For this review, take the finished solid that the model builds, in its own axes (mm). Round coordinates to 2 decimals unless told otherwise and drop trailing zeros. Order: outer loops, then holes, each group sorted by start corner. A loop starts at its lowest first (then second) coordinate and runs counter-clockwise, first axis right, second up.
```python
from build123d import *

# Parameters (mm, degrees)
F1_DEPTH = 3
F2_D     = 3.3
F3_D     = 4.3
F4_R     = 5


# Not quite as in the source:
# - a feature names something its author has since deleted; it is built from what else it names


with BuildPart() as f1:
    # F0 (on Top) → F1 (new body)
    with BuildSketch(Plane.XY):
        Polygon((-43.9476147294, -54.0188625455), (24.4538411498, -54.0188625455), (24.4538411498, 61.4031404257), (-43.9476147294, 61.4031404257), (-43.9476147294, 45.1967306435), align=None)
    extrude(amount=F1_DEPTH)

    # F2 (through all)
    with Locations(Plane(origin=(0, 0, 0), x_dir=(1, 0, 0), z_dir=(0, 0, -1))):
        with Locations((-37.0104938323, -45.9071589798), (11.4895061677, -52.6071589798), (11.4895061677, 30.2928410202), (-37.0104938323, 28.9928410202)):
            Hole(F2_D / 2)

    # F3 (through all)
    with Locations(Plane(origin=(0, 0, 0), x_dir=(1, 0, 0), z_dir=(0, 0, -1))):
        with Locations((-21.5, -46.5), (21.5, -46.5), (21.5, 46.5), (-21.5, 46.5)):
            Hole(F3_D / 2)

    # F4
    f4_edges = [f1.edges().sort_by_distance(p)[0] for p in [
        (-43.947615, -54.018863, 1.5),
        (24.453841, -54.018863, 1.5),
        (-43.947615, 61.40314, 1.5),
        (24.453841, 61.40314, 1.5),
    ]]
    fillet(f4_edges, radius=F4_R)


solid = f1.part
```
Q1. Wall thickness on line 1 (X direction, y = -46.5, z = 2.15); line 2 (Y direction, x = -21.5, z = 2.15); line 3 (Y direction, x = 21.5, z = 1.4): over which ranges is each line inside the solid? List them lowest first.
Q2. Mouldability with a two-part tool opening along Y and no side actions: class faces 1 (the face through (11.847, -28.682, 1.521)), 2 (the face through (-10, 5, 3)), 3 (the face through (-10, -54.019, 1)) as +Y half, -Y half, draft (parallel to the pull), parting line (faces both ways), or undercut.
Q3. Take a section at A-A, the plane x = -21.5. State the section outline as (y, z) points, plus the area to 3 significant figures.
Q4. Take a section at B-B, the plane x = 21.5. State the section outline as (y, z) points.
Working result:
1. line 1: x = -43.95 to -23.65, -19.35 to 19.35, 23.65 to 24.45
1. line 2: y = -54.02 to -48.65, -44.35 to 44.35, 48.65 to 61.4
1. line 3: y = -53.58 to -48.65, -44.35 to 44.35, 48.65 to 60.97
2. face 1: undercut
2. face 2: draft
2. face 3: -Y half
3. outline: (-54.02, 0) - (-48.65, 0) - (-48.65, 3) - (-54.02, 3) - close; (-44.35, 0) - (44.35, 0) - (44.35, 3) - (-44.35, 3) - close; (48.65, 0) - (61.4, 0) - (61.4, 3) - (48.65, 3) - close
3. area: 320 mm2
4. outline: (-53.58, 0) - (-48.65, 0) - (-48.65, 3) - (-53.58, 3) - close; (-44.35, 0) - (44.35, 0) - (44.35, 3) - (-44.35, 3) - close; (48.65, 0) - (60.97, 0) - (60.97, 3) - (48.65, 3) - close
